Could you check a few things on this model? Use its own coordinates, in mm. A direction names the side the tool comes from. Coordinates: 2 decimals unless noted, no trailing zeros. Loops run counter-clockwise (first coordinate to the right, second up) from the corner with the lowest first, then second, coordinate; pieces in that order, holes last. Notation, with made-up numbers: (-34, -12.5) -> (21, -12.5) arc R10 ccw to (21, 6.5) -> close; hole circle Ø6 at (55, 57.5). An arc over 180 degrees is marked (long way). One line per question, with ' | ' between items.
from build123d import *

# Parameters (mm, degrees)
F0_W     = 50.8
F0_H     = 76.2
F1_DEPTH = 76.2
F2_W     = 76.2
F2_H     = 38.1
F3_DEPTH = 50.8
F4_W     = 76.2
F4_H     = 20.904989
F5_DEPTH = 25.4


with BuildPart() as f1:
    # F0 (on Front) → F1 (new body)
    with BuildSketch(Plane.XZ):
        with Locations((-25.4, 38.1)):
            Rectangle(F0_W, F0_H)
    extrude(amount=F1_DEPTH)

    # F2 (on face) → F3 (join)
    with BuildSketch(Plane.YZ):
        with Locations((-38.1, 19.05)):
            Rectangle(F2_W, F2_H)
    extrude(amount=F3_DEPTH)

    # F4 (on face) → F5 (join)
    with BuildSketch(Plane.YZ):
        with Locations((-38.1, 48.552494)):
            Rectangle(F4_W, F4_H)
    extrude(amount=F5_DEPTH)


solid = f1.part
1) If we section it at B-B on z = 65.5: Please give me the cut outline in (x, y), and give its area (3 significant figures).
Data:
outline: (-50.8, -76.2) -> (0, -76.2) -> (0, 0) -> (-50.8, 0) -> close | area: 3,870 mm²
2) I'm going to push flat-ended pins straight in: pin 1 Ø4 at (x, y) = (-2, -31) entering from -Z; pin 2 Ø14 at (y, z) = (-20, 68) entering from +X; pin 3 Ø6.5 at (y, z) = (-26, 53) entering from +X; pin 4 Ø20.5 at (x, y) = (38.5, -40) entering from +Z. Where does each tip first touch, or does it pass through?
Data:
pin 1: z = 0 | pin 2: x = 0 | pin 3: x = 25.4 | pin 4: z = 38.1
3) If we section it at A-A on y = -11: Please give me the cut outline in (x, z), and give its area (3 significant figures).
Data:
outline: (-50.8, 0) -> (50.8, 0) -> (50.8, 38.1) -> (25.4, 38.1) -> (25.4, 59) -> (0, 59) -> (0, 76.2) -> (-50.8, 76.2) -> close | area: 6,340 mm²
4) If we section it at C-C on z = 51: Please give me the cut outline in (x, y).
Data:
outline: (-50.8, -76.2) -> (25.4, -76.2) -> (25.4, 0) -> (-50.8, 0) -> close
5) I need wall thicknesses on line 1 along Z through (x, y) = (43, -5); line 2 along Z through (x, y) = (15, -53.5); line 3 along X through (y, z) = (-65.5, 67). Which ranges of each line are inside material? Lowest first, please. Write a range as from..to.
Data:
line 1: 0..38.1 | line 2: 0..59 | line 3: -50.8..0
6) On a 3-axis mill with a long thin cutter (end or side, diameter ignored), from which of +Z, -Z, +X, -X, +Y, -Y can I reach the whole of each face in a straight line? I mean faces 1 (the face through (13, -39, 59.005)), 2 (the face through (-1, -39, 0)). Say none if no direction works.
Data:
face 1: +Z, +X, +Y, -Y | face 2: -Z, +X, -X, +Y, -Y
